Geometry: final body of the model. Coordinates: model frame, mm. Give positions to 0.01 mm unless a question says otherwise; leave off trailing zeros. Write each loop counter-clockwise with the first axis right and the second up, starting at its lowest first coordinate (ties: lowest second). Pieces come first, ordered by that corner, then holes. Notation, with made-up numbers: M 45,-35 L 67,-35 A21 cw 67,-7 Z; hole C 24,50 d8. An arc over 180 degrees is marked long. Use a Markdown table: item, result. Add a question column.
1) Section C-C on y = -12.7. Return the cut outline in (x, z), then the cut area to 3 significant figures.
2) Line query: line 1 (X direction, y = -12, z = 42); line 2 (X direction, y = -12.7, z = 56.5); line 3 (Y direction, x = 12, z = 58). Output: solid intervals per line, ascending.
3) Section D-D on x = -11. Return the cut outline in (y, z), then the cut area to 3 significant figures.
4) Section B-B on z = 30. Return the cut outline in (x, y).
5) Section A-A on x = 12.7. Return the cut outline in (y, z), then the cut area to 3 significant figures.
6) Draft query along Y for faces 1 (the flat face through (25.4, -8, 58)), 2 (the flat face through (12.53, -1.93, 1.88)), 3 (the conical face through (13.76, -9.34, 2.38)). Return one class per face: +Y half, -Y half, draft (parallel to the pull), parting line (faces both ways), or undercut.
7) Pin query (flat end, axial travel): pin 1 (9 mm diameter, centred on x = 12.7, y = -12.7, fed in from +Z); pin 2 (6 mm diameter, centred on x = -3.5, z = 78.5, fed in from +Y); pin 3 (1.5 mm diameter, centred on x = -8, z = 48, fed in from +Y). Return the tip coordinate at first contact, or that it passes through.
```python
from build123d import *

# Parameters (mm, degrees)
SKETCH1_W           = 114.3
SKETCH1_H           = 50.8
BOSS_EXTRUDE1_DEPTH = 25.4
SKETCH2_R           = 3.3655
CUT_EXTRUDE1_DEPTH  = 128.633420388
CHAMFER1_SIZE       = 2.54
BOSS_EXTRUDE2_DEPTH = 114.3
CHAMFER2_SIZE       = 3.81
FILLET1_R           = 6.35


with BuildPart() as part:
    # Sketch1 → Boss-Extrude1 (new body)
    with BuildSketch(Plane(origin=(0, 0, 0), x_dir=(0, 0, -1), z_dir=(1, 0, 0))):
        with Locations((-57.15, -25.4)):
            Rectangle(SKETCH1_W, SKETCH1_H)
    extrude(amount=BOSS_EXTRUDE1_DEPTH)

    # Sketch2 → Cut-Extrude1 (cut, through all)
    with BuildSketch(Plane(origin=(0, 0, 0), x_dir=(-1, 0, 0), z_dir=(0, 0, -1))):
        with Locations(Location((-12.7, -12.7, 0), (0, 0, 90))):
            Circle(SKETCH2_R)
    extrude(amount=-CUT_EXTRUDE1_DEPTH, mode=Mode.SUBTRACT)

    # Chamfer1
    chamfer1_edges = [part.edges().sort_by_distance(p)[0] for p in [
        (12.7, -16.0655, 114.3),
        (12.7, -16.0655, 0),
    ]]
    chamfer(chamfer1_edges, length=CHAMFER1_SIZE)

    # Sketch3 → Boss-Extrude2 (add)
    with BuildSketch(Plane(origin=(0, 0, 0), x_dir=(-1, 0, 0), z_dir=(0, 0, -1))):
        Polygon((-50.8, -44.45), (-25.4, -12.7), (-25.4, -50.8), (-50.8, -50.8), align=None)
        Polygon((25.4, -50.8), (25.4, -44.45), (0, -12.7), (0, -50.8), align=None)
    extrude(amount=-BOSS_EXTRUDE2_DEPTH)

    # Chamfer2
    chamfer2_edges = [part.edges().sort_by_distance(p)[0] for p in [
        (12.7, 0, 114.3),
        (12.7, 0, 0),
    ]]
    chamfer(chamfer2_edges, length=CHAMFER2_SIZE)

    # Fillet1
    fillet1_edges = [part.edges().sort_by_distance(p)[0] for p in [
        (-25.4, -44.45, 57.15),
        (0, -12.7, 57.15),
        (0, 0, 57.15),
        (25.4, 0, 57.15),
        (50.8, -44.45, 57.15),
        (25.4, -12.7, 57.15),
    ]]
    fillet(fillet1_edges, radius=FILLET1_R)


solid = part.part
```
Found:
| question | item | result |
|---|---|---|
| 1 | outline | M -0.4,0 L 6.79,0 L 9.33,2.54 L 9.33,111.76 L 6.79,114.3 L -0.4,114.3 Z; M 16.07,2.54 L 18.61,0 L 25.8,0 L 25.8,114.3 L 18.61,114.3 L 16.07,111.76 Z |
| 1 | area | 2,210 mm² |
| 2 | line 1 | -0.19 to 9.41, 15.99 to 25.59 |
| 2 | line 2 | -0.4 to 9.33, 16.07 to 25.8 |
| 2 | line 3 | -50.8 to -15.99, -9.41 to 0 |
| 3 | outline | M -50.8,0 L -26.45,0 L -26.45,114.3 L -50.8,114.3 Z |
| 3 | area | 2,780 mm² |
| 4 | outline | M -25.4,-50.8 L 50.8,-50.8 L 50.8,-46.68 A6.35 ccw 49.41,-42.71 L 26.79,-14.44 A6.35 cw 25.4,-10.47 L 25.4,-6.35 A6.35 ccw 19.05,0 L 6.35,0 A6.35 ccw 0,-6.35 L 0,-10.47 A6.35 cw -1.39,-14.44 L -24.01,-42.71 A6.35 ccw -25.4,-46.68 Z; hole C 12.7,-12.7 d6.73 |
| 5 | outline | M -50.8,0 L -18.61,0 L -16.07,2.54 L -16.07,111.76 L -18.61,114.3 L -50.8,114.3 Z; M -9.33,2.54 L -6.79,0 L -3.81,0 L 0,3.81 L 0,110.49 L -3.81,114.3 L -6.79,114.3 L -9.33,111.76 Z |
| 5 | area | 5,010 mm² |
| 6 | face 1 | draft |
| 6 | face 2 | +Y half |
| 6 | face 3 | undercut |
| 7 | pin 1 | z = 112.89 |
| 7 | pin 2 | y = -12.94 |
| 7 | pin 3 | y = -21.76 |
